```python
from build123d import *

# Parameters (mm, degrees)
ESQUISSE1_W             = 22
ESQUISSE1_H             = 23
BOSS_EXTRU_1_DEPTH      = 6.1
BOSS_EXTRU_2_DEPTH      = 4.5
ESQUISSE3_R             = 2.45
BOSS_EXTRU_3_DEPTH      = 2.8
ESQUISSE4_W             = 2.5
ESQUISSE4_H             = 4.75
BOSS_EXTRU_4_DEPTH      = 6.1
ENL_V_MAT_EXTRU_1_REACH = 21
ESQUISSE5_R             = 0.75


with BuildPart() as part:
    # Esquisse1 → Boss.-Extru.1 (new body, symmetric)
    with BuildSketch(Plane(origin=(0, 0, 0), x_dir=(0, 0, -1), z_dir=(1, 0, 0))):
        Rectangle(ESQUISSE1_W, ESQUISSE1_H)
    extrude(amount=BOSS_EXTRU_1_DEPTH, both=True)

    # Esquisse2 → Boss.-Extru.2 (add)
    with BuildSketch(Plane.XY.offset(11)):
        with BuildLine():
            ThreePointArc((2.749629517, -0.045138889), (0, 11.5), (-2.749629517, -0.045138889))
            ThreePointArc((-2.749629517, -0.045138889), (0, -2.75), (2.749629517, -0.045138889))
        make_face()
    extrude(amount=BOSS_EXTRU_2_DEPTH)

    # Esquisse3 → Boss.-Extru.3 (add)
    with BuildSketch(Plane.XY.offset(15.5)):
        with Locations((0, 5.4)):
            Circle(ESQUISSE3_R)
    extrude(amount=BOSS_EXTRU_3_DEPTH)

    # Esquisse4 → Boss.-Extru.4 (add, symmetric)
    with BuildSketch(Plane(origin=(0, 0, 0), x_dir=(0, 0, -1), z_dir=(1, 0, 0))):
        with Locations((-6.75, 13.875)):
            Rectangle(ESQUISSE4_W, ESQUISSE4_H)
        with Locations((-6.75, -13.875)):
            Rectangle(ESQUISSE4_W, ESQUISSE4_H)
    extrude(amount=BOSS_EXTRU_4_DEPTH, both=True)

    # Esquisse5 → Enlèv. mat.-Extru.1 (cut, up to next)
    with BuildSketch(Plane.XY.offset(8), mode=Mode.PRIVATE) as enl_v_mat_extru_1_sk1:
        with Locations((0, 13.875)):
            Circle(ESQUISSE5_R)
    enl_v_mat_extru_1_tool1 = extrude(enl_v_mat_extru_1_sk1.sketch, amount=-ENL_V_MAT_EXTRU_1_REACH, mode=Mode.PRIVATE) & part.part
    add(enl_v_mat_extru_1_tool1.solids().sort_by_distance((0, 13.875, 8))[0], mode=Mode.SUBTRACT)
    # Esquisse5 → Enlèv. mat.-Extru.1 (cut, up to next)
    with BuildSketch(Plane.XY.offset(8), mode=Mode.PRIVATE) as enl_v_mat_extru_1_sk2:
        with Locations((0, -13.875)):
            Circle(ESQUISSE5_R)
    enl_v_mat_extru_1_tool2 = extrude(enl_v_mat_extru_1_sk2.sketch, amount=-ENL_V_MAT_EXTRU_1_REACH, mode=Mode.PRIVATE) & part.part
    add(enl_v_mat_extru_1_tool2.solids().sort_by_distance((0, -13.875, 8))[0], mode=Mode.SUBTRACT)


solid = part.part
```
Here's how the part is built. I have some questions about the finished solid (model axes, mm). A direction names the side the tool comes from. Round coordinates to 2 decimals unless told otherwise and drop trailing zeros. Loops run counter-clockwise (first coordinate to the right, second up) from the corner with the lowest first, then second, coordinate; pieces in that order, holes last.
1. Suppose I cut it at D-D, the plane x = -4.5. Please give me the cut outline in (y, z).
Answers:
outline: (-16.25, 5.5) - (-11.5, 5.5) - (-11.5, -11) - (11.5, -11) - (11.5, 5.5) - (16.25, 5.5) - (16.25, 8) - (11.5, 8) - (11.5, 11) - (9.52, 11) - (9.52, 15.5) - (1.28, 15.5) - (1.28, 11) - (-11.5, 11) - (-11.5, 8) - (-16.25, 8) - close
2. Suppose I cut it at B-B, the plane y = 12. Please give me the cut outline in (x, z).
Answers:
outline: (-6.1, 5.5) - (6.1, 5.5) - (6.1, 8) - (-6.1, 8) - close
3. Thinking about a two-plate mould opening in X: for faces 1 (the face through (-0.1, 14.62, 6.77)), 2 (the face through (0.228, 11.496, 13.218)), 3 (the face through (-6.1, 0, 0)), 4 (the face through (0, -11.5, 10)), which applies, released by +X, released by -X, zero draft, split by the parting line, or undercut?
Answers:
face 1: undercut
face 2: split by the parting line
face 3: released by -X
face 4: zero draft
4. For faces 5 (the face through (0.1, -12.9, 5.5)), 6 (the face through (-0.5, 3, 16.9)), 7 (the face through (0, 15, 5.5)), 8 (the face through (0, 15, 8)), 9 (the face through (-5, 10, 11)), which set-ups out of +Z, -Z, +X, -X, +Y, -Y let a thin tool reach every point of the face, with its end or its side?
Answers:
face 5: -Z, +X, -X, -Y
face 6: +Z
face 7: -Z, +X, -X, +Y
face 8: +Z, +X, -X, +Y
face 9: +Z, -X, +Y
5. Will these pins go through, and if not, where does the flat tip stop? pin 1 (2 mm diameter, centred on x = -2, z = -3, fed in from -Y); pin 2 (1.5 mm diameter, centred on x = 2, y = 2, fed in from +Z); pin 3 (0.9 mm diameter, centred on x = 0.5, z = 9, fed in from +Y).
Answers:
pin 1: stops at y = -11.5
pin 2: stops at z = 15.5
pin 3: stops at y = 11.5
6. Suppose I cut it at C-C, the plane z = 9.25. Please give me the cut outline in (x, y), and give its area (3 significant figures).
Answers:
outline: (-6.1, -11.5) - (6.1, -11.5) - (6.1, 11.5) - (-6.1, 11.5) - close
area: 281 mm2
7. Suppose I cut it at A-A, the plane x = 1.5. Please give me the cut outline in (y, z), and give its area (3 significant figures).
Answers:
outline: (-16.25, 5.5) - (-11.5, 5.5) - (-11.5, -11) - (11.5, -11) - (11.5, 5.5) - (16.25, 5.5) - (16.25, 8) - (11.5, 8) - (11.5, 11) - (11.31, 11) - (11.31, 15.5) - (7.34, 15.5) - (7.34, 18.3) - (3.46, 18.3) - (3.46, 15.5) - (-2.3, 15.5) - (-2.3, 11) - (-11.5, 11) - (-11.5, 8) - (-16.25, 8) - close
area: 602 mm2
8. If I drill on probe 1 along Y at (x, z) = (0, 6.3) (3 decimals); probe 2 along Z at (x, y) = (-1.25, 13.5); probe 3 along Y at (x, z) = (2.25, 8.5), over which ranges is the centre line in solid material (lowest first)?
Answers:
probe 1: y = -16.25 to -14.625, -13.125 to 13.125, 14.625 to 16.25
probe 2: z = 5.5 to 8
probe 3: y = -11.5 to 11.5
